Input: part model. Units: mm. Frame: model coordinates. Face numbers are marked on the shaded views. A direction names the side the tool comes from. Coordinates: 2 decimals unless noted, no trailing zeros. Loops run counter-clockwise (first coordinate to the right, second up) from the corner with the lowest first, then second, coordinate; pieces in that order, holes last.
(1) Section B-B, the plane x = 29. Return loops of the section in (y, z).
(2) Mould query, pull axis X, two halves, no side actions, for the marked faces 3, 4, 5 and 6. Classes: released by +X, released by -X, zero draft, split by the parting line, or undercut.
(3) Section A-A, the plane x = 0. Give the number of separate pieces and of enclosed holes in the cut face, then the cut area to 3 significant figures.
(4) Line query: L1, parallel to Y at x = 0, z = 2.9; L2, parallel to X at y = 25, z = 9.5; L3, parallel to X at y = 6, z = 2.75. Output: solid intervals per line, ascending.
(5) Set-up query: the marked faces 1 and 2. Return all of +Z, -Z, +X, -X, +Y, -Y with unobstructed straight access to the full face (end or side cutting, diameter ignored); none if empty.
(6) Contact query for flat-ended pins moving along their axis: P1, Ø18, axis at x = 20.5, y = 7, coming from the +Z side; P2, Ø1.9, axis at x = 40.5, y = -0.5, coming from the +Z side; P3, Ø0.6, axis at y = 19.5, z = 9.5, coming from the +X side; P4, Ø1.8, axis at x = 0, y = 0, coming from the -Z side. Output: stop coordinate, or through.
(7) Section C-C, the plane z = 7.5. Return loops of the section in (x, y), then the cut area to 3 significant figures.
```python
from build123d import *

# Parameters (mm, degrees)
EXTRUDE003_DEPTH = 2
SKETCH001_W      = 57.0675
SKETCH001_H      = 36.03
SKETCH001_R      = 1.5
EXTRUDE001_DEPTH = 2
SKETCH006_W      = 57.0675
SKETCH006_H      = 36.03
EXTRUDE006_DEPTH = 2
EXTRUDE002_DEPTH = 5
CHAMFER001_SIZE  = 1


with BuildPart() as obj1:
    # Sketch003 → Extrude003 (new body)
    with BuildSketch(Plane.XY.offset(9)):
        Polygon((-11.59465, 29.4474), (43.47285, 29.4474), (43.47285, -4.5826), (-11.59465, -4.5826), (-11.59465, 5.4324), (-10.59465, 5.4324), (-10.59465, -3.5826), (42.47285, -3.5826), (42.47285, 28.4474), (-10.59465, 28.4474), (-10.59465, 19.4324), (-11.59465, 19.4324), align=None)
    extrude(amount=EXTRUDE003_DEPTH)


with BuildPart() as obj2:
    # Sketch001 → Extrude001 (new body)
    with BuildSketch(Plane.XY.offset(2)):
        with Locations((15.9391, 12.4324)):
            Rectangle(SKETCH001_W, SKETCH001_H)
        with Locations((0.00035, 24.9999)):
            Circle(SKETCH001_R, mode=Mode.SUBTRACT)
        with Locations((39.00035, 24.9999)):
            Circle(SKETCH001_R, mode=Mode.SUBTRACT)
        with Locations((39.00035, -0.0001)):
            Circle(SKETCH001_R, mode=Mode.SUBTRACT)
        Circle(SKETCH001_R, mode=Mode.SUBTRACT)
        with BuildLine():
            Line((-10.59465, 28.4474), (-2.9993, 28.4474))
            Line((-2.9993, 28.4474), (-2.9993, 24.9999))
            ThreePointArc((-2.9993, 24.9999), (-0.777953, 22.102712), (2.5965, 23.495965))
            ThreePointArc((3, 24.9999), (2.417325, 24.350133), (2.5965, 23.495965))
            Line((3, 24.9999), (3, 28.4474))
            Line((3, 28.4474), (36.00035, 28.4474))
            Line((36.00035, 24.9999), (36.00035, 28.4474))
            ThreePointArc((36.00035, 24.9999), (36.87903, 22.87858), (39.00035, 21.9999))
            Line((42.47285, 21.9999), (39.00035, 21.9999))
            Line((42.47285, 21.9999), (42.47285, 2.9999))
            Line((42.47285, 2.9999), (39.00035, 2.9999))
            ThreePointArc((39.00035, 2.9999), (36.87903, 2.12122), (36.00035, -0.0001))
            Line((36.00035, -0.0001), (36.00035, -3.5826))
            Line((36.00035, -3.5826), (3, -3.5826))
            Line((3, 0), (3, -3.5826))
            ThreePointArc((3, 0), (0, 3), (-3, 0))
            Line((-3, -3.5826), (-3, 0))
            Line((-3, -3.5826), (-10.59465, -3.5826))
            Line((-10.59465, -3.5826), (-10.59465, 28.4474))
        make_face(mode=Mode.SUBTRACT)
    extrude(amount=EXTRUDE001_DEPTH)


with BuildPart() as base:
    # Sketch006 → Extrude006 (new body)
    with BuildSketch(Plane.XY):
        with Locations((15.9391, 12.4324)):
            Rectangle(SKETCH006_W, SKETCH006_H)
        Polygon((41.996992, 24.857996), (40.621563, 27.524116), (37.624921, 27.66602), (36.003708, 25.141804), (37.379137, 22.475684), (40.375779, 22.33378), align=None, mode=Mode.SUBTRACT)
        Polygon((3.00035, 24.9999), (1.50035, 27.597976), (-1.49965, 27.597976), (-2.99965, 24.9999), (-1.49965, 22.401824), (1.50035, 22.401824), align=None, mode=Mode.SUBTRACT)
        Polygon((3, 0), (1.5, 2.598076), (-1.5, 2.598076), (-3, 0), (-1.5, -2.598076), (1.5, -2.598076), align=None, mode=Mode.SUBTRACT)
        Polygon((36.00035, 0), (37.500263, -2.598126), (40.500263, -2.598226), (42.00035, -0.0002), (40.500437, 2.597926), (37.500437, 2.598026), align=None, mode=Mode.SUBTRACT)
    extrude(amount=EXTRUDE006_DEPTH)


with BuildPart() as fusion002:
    # Sketch002 → Extrude002 (new body)
    with BuildSketch(Plane.XY.offset(4)):
        Polygon((-10.59465, 28.4474), (42.47285, 28.4474), (42.47285, -3.5826), (-10.59465, -3.5826), (-10.59465, 5.4324), (-12.59465, 5.4324), (-12.59465, -5.5826), (44.47285, -5.5826), (44.47285, 30.4474), (-12.59465, 30.4474), (-12.59465, 19.4324), (-10.59465, 19.4324), align=None)
    extrude(amount=EXTRUDE002_DEPTH)

    # Fusion: union obj2, BASE
    add(obj2.part)
    add(base.part)

    # Chamfer001
    chamfer001_edges = [fusion002.edges().sort_by_distance(p)[0] for p in [
        (15.9391, 30.4474, 0),
        (44.47285, 12.4324, 0),
        (15.9391, -5.5826, 0),
        (-12.59465, 12.4324, 0),
        (-12.59465, 30.4474, 4.5),
        (-12.59465, -5.5826, 4.5),
        (44.47285, -5.5826, 4.5),
        (44.47285, 30.4474, 4.5),
    ]]
    chamfer(chamfer001_edges, length=CHAMFER001_SIZE)

    # Fusion002: union obj1
    add(obj1.part)


solid = fusion002.part
```
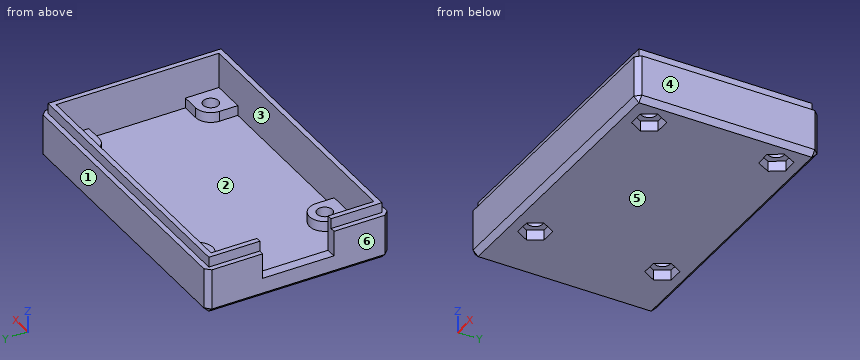
Report:
1. outline: (-5.58, 1) - (-4.58, 0) - (29.45, 0) - (30.45, 1) - (30.45, 9) - (29.45, 9) - (29.45, 11) - (28.45, 11) - (28.45, 2) - (-3.58, 2) - (-3.58, 11) - (-4.58, 11) - (-4.58, 9) - (-5.58, 9) - close
2. face 3: undercut
2. face 4: released by +X
2. face 5: zero draft
2. face 6: released by -X
3. separate pieces: 3
3. enclosed holes: 0
3. area: 96.3 mm2
4. L1: y = -5.58 to -1.5, 1.5 to 3, 22 to 23.5, 26.5 to 30.45
4. L2: x = -11.59 to -10.59, 42.47 to 43.47
4. L3: x = -12.59 to -10.59, 42.47 to 44.47
5. face 1: +Z, -Z, +X, -X, +Y
5. face 2: +Z
6. P1: stops at z = 2
6. P2: stops at z = 4
6. P3: stops at x = 43.47
6. P4: passes through
7. outline: (-12.59, -4.58) - (-11.59, -5.58) - (43.47, -5.58) - (44.47, -4.58) - (44.47, 29.45) - (43.47, 30.45) - (-11.59, 30.45) - (-12.59, 29.45) - (-12.59, 19.43) - (-10.59, 19.43) - (-10.59, 28.45) - (42.47, 28.45) - (42.47, -3.58) - (-10.59, -3.58) - (-10.59, 5.43) - (-12.59, 5.43) - close
7. area: 326 mm2
